Could you check a few things on this drawing? It's one solid part, dimensions in mm from its lowest x, y, z. A direction names the side the tool comes from. Give positions to 0.01 mm unless a question says otherwise; leave off trailing zeros. Loops run counter-clockwise (first coordinate to the right, second up) from the corner with the lowest first, then second, coordinate; pieces in that order, holes last. Notation, with made-up numbers: M 11,62 L 57,62 A20 ccw 57,88 Z; hole C -18.5,1.5 d8. An arc over 180 degrees is marked long. Answer in a Markdown table with one row per item. Add a question column.
1. Thinking about a two-plate mould opening in X: for the marked faces 3, 4 and 5, which applies, released by +X, released by -X, zero draft, split by the parting line, or undercut?
2. If we section it at A-A on x = 11: List the corners of the cut face in (y, z) for me.
3. I need wall thicknesses on line 1 along X through (y, z) = (14, 2.5); line 2 along Z through (x, y) = (17, 9.5); line 3 along Z through (x, y) = (12, 15.25). Which ranges of each line are inside material? Lowest first, please. Write a range as from..to.
4. I'm going to push flat-ended pins straight in: pin 1 Ø2 at (x, y) = (11, 8.5) entering from +Z; pin 2 Ø6 at (x, z) = (15.5, 2.5) entering from +Y. Where does each tip first touch, or does it pass through?
5. If we section it at B-B on z = 6.25: List the corners of the cut face in (x, y) for me.
6. Which directions (+Z, -Z, +X, -X, +Y, -Y) give clear straight access to the entire face, cutting with the end or side of a thin tool? Please do the marked faces 1 and 2.
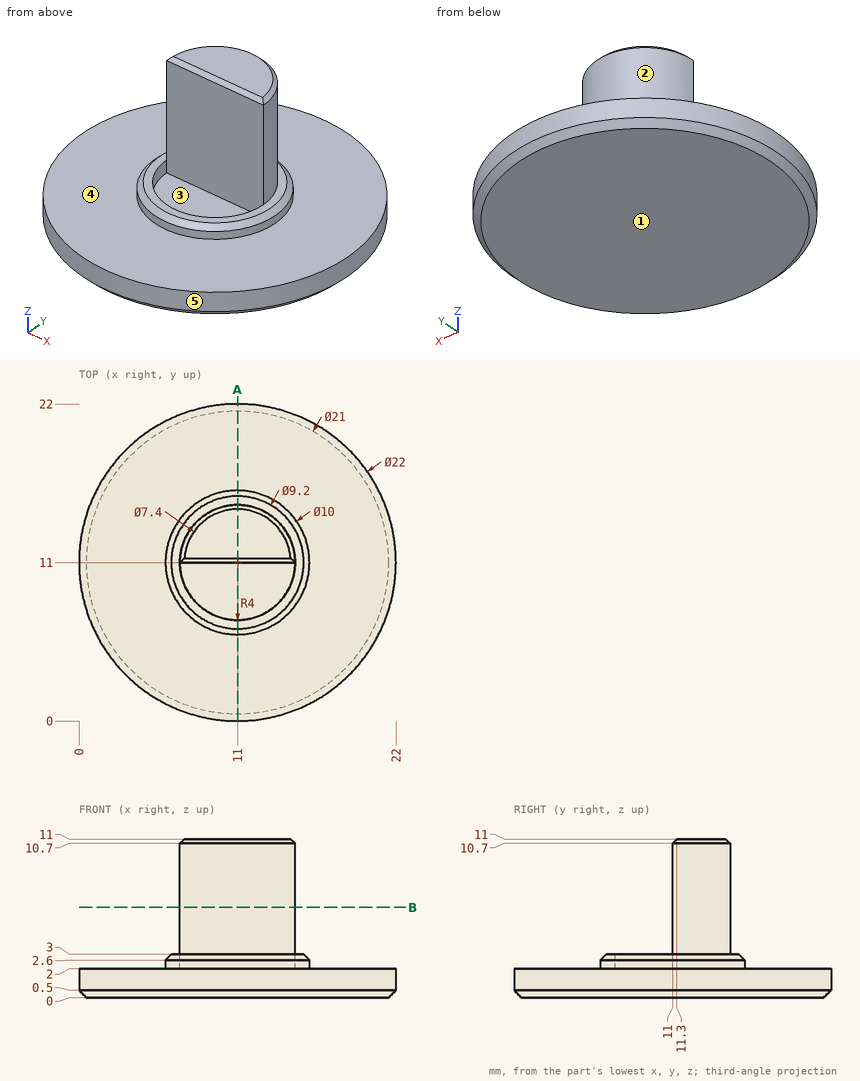
Results:
| question | item | result |
|---|---|---|
| 1 | face 3 | undercut |
| 1 | face 4 | zero draft |
| 1 | face 5 | split by the parting line |
| 2 | outline | M 0,0.5 L 0.5,0 L 21.5,0 L 22,0.5 L 22,2 L 16,2 L 16,2.6 L 15.6,3 L 15,3 L 15,10.7 L 14.7,11 L 11.3,11 L 11,10.7 L 11,2 L 7,2 L 7,3 L 6.4,3 L 6,2.6 L 6,2 L 0,2 Z |
| 3 | line 1 | 7..15 |
| 3 | line 2 | 0..2 |
| 3 | line 3 | 0..3 |
| 4 | pin 1 | z = 2 |
| 4 | pin 2 | y = 21.89 |
| 5 | outline | M 7,11 L 15,11 A4 ccw Z |
| 6 | face 1 | -Z, +X, -X, +Y, -Y |
| 6 | face 2 | +Z, +Y |
